Geometry: final body of the model. Coordinates: model frame, mm. Give positions to 0.01 mm unless a question says otherwise; leave off trailing zeros. Loops run counter-clockwise (first coordinate to the right, second up) from the corner with the lowest first, then second, coordinate; pieces in that order, holes last. Notation, with made-up numbers: M 22,14 L 33,14 A25 cw 33,33 Z; hole C -1,46.25 d5. An arc over 180 degrees is marked long. Put each result on its own line as item: value.
```python
from build123d import *

# Parameters (mm, degrees)
SKETCH1_R           = 92.075
BOSS_EXTRUDE1_DEPTH = 101.6
SHELL1_T            = -7.9375


with BuildPart() as part:
    # Sketch1 → Boss-Extrude1 (new body)
    with BuildSketch(Plane.XY):
        Circle(SKETCH1_R)
    extrude(amount=BOSS_EXTRUDE1_DEPTH)

    # Sketch2 → Revolve1 (revolve)
    with BuildSketch(Plane(origin=(0, 0, 0), x_dir=(0, 0, -1), z_dir=(1, 0, 0))):
        with BuildLine():
            Line((0, 0), (38.1, 0))
            ThreePointArc((38.1, 0), (28.198839221, 49.823226574), (0, 92.075))
            Line((0, 92.075), (0, 0))
        make_face()
    revolve(axis=Axis((0, 0, 0), (0, 0, -1)))

    # Shell1
    shell1_openings = [part.faces().sort_by_distance(p)[0] for p in [
        (0, 0, 101.6),
    ]]
    offset(amount=SHELL1_T, openings=shell1_openings)


solid = part.part
```
Item 1: Line query: probe 1 along X at (y, z) = (0, 78) (1 decimal); probe 2 along Y at (x, z) = (9, 42). Output: solid intervals per line, ascending. Write a range as [from, to].
Output values:
probe 1: [-92.1, -84.1], [84.1, 92.1]
probe 2: [-91.63, -83.65], [83.65, 91.63]
Item 2: Section D-D on x = 67.5. Output: boundary loops of the cut face in (y, z).
Output values:
outline: M -62.62,0 A111.46 ccw 62.62,0 L 62.62,101.6 L 50.23,101.6 L 50.23,3.35 A102.07 cw -50.23,3.35 L -50.23,101.6 L -62.62,101.6 Z
Item 3: Mould query, pull axis X, two halves, no side actions, for faces 1 (the flat face through (40, -75, 101.6)), 2 (the cylindrical face through (-18.239, -82.137, 51.788)), 3 (the cylindrical face through (-73.068, -56.026, 50.089)). Classes: pulls with the +X half, pulls with the -X half, needs draft (parallel to the pull), parting line crosses it, or undercut.
Output values:
face 1: needs draft
face 2: undercut
face 3: parting line crosses it
Item 4: Section A-A on x = 0. Output: boundary loops of the cut face in (y, z) (1 decimal).
Output values:
outline: M -92.1,0 A130.3 ccw 92.1,0 L 92.1,101.6 L 84.1,101.6 L 84.1,3.4 A122.4 cw -84.1,3.4 L -84.1,101.6 L -92.1,101.6 Z
Item 5: Pin query (flat end, axial travel): pin 1 Ø3 at (y, z) = (69, 26.5) entering from +X; pin 2 Ø8 at (y, z) = (38.5, 49) entering from +X; pin 3 Ø10 at (y, z) = (7.5, -1.5) entering from -X. Return the tip coordinate at first contact, or that it passes through.
Output values:
pin 1: x = 62.62
pin 2: x = 85.37
pin 3: x = -92.03
